Read the model definition and answer for the solid it produces. Units are mm, in the model's axes. Give positions to 0.01 mm unless a question says otherwise; leave off trailing zeros. Loops run counter-clockwise (first coordinate to the right, second up) from the corner with the lowest first, then second, coordinate; pieces in that order, holes last. Notation, with made-up numbers: (-36, 43.5) - (9, 43.5) arc R30 cw to (9, 69.5) - close; hole circle Ø11 at (69, 80.25). An arc over 180 degrees is marked (long way). Use a Markdown table: item, result. Add a question column.
Item 1: Consider probe 1 along X at (y, z) = (61.5, -12.25); probe 2 along X at (y, z) = (28, -13); probe 3 along Z at (x, y) = (4.5, 49). Determine where each line is inside the solid, lowest interval first. Write a range as [from, to].
Item 2: A cutting plane is placed at C-C (x = 0). Determine the outline of the cut face in (y, z).
Item 3: A cutting plane is placed at B-B (y = 37.5). Determine the outline of the cut face in (x, z).
Item 4: A cutting plane is placed at D-D (z = 12). Determine the outline of the cut face in (x, y), plus the area to 3 significant figures.
Item 5: A cutting plane is placed at A-A (z = 7). Determine the outline of the cut face in (x, y).
Autodesk Fusion 360 part; units mm, degrees
sketch "Sketch1" plane through (0, 0, 0) normal (0, 0, 1) x (1, 0, 0)
sketch "Sketch2" plane through (0, 0, 0) normal (0, 1, 0) x (1, 0, 0)
  line L0 (24, -15) -> (-24, -15)
  line L1 (-24, -15) -> (-24, 15)
  line L2 (-24, 15) -> (24, 15)
  line L3 (24, 15) -> (24, -15)
  line L4 (24, -15) -> (-24, 15) construction
  line L5 (-24, -15) -> (24, 15) construction
  dimension "d3" = 48
  dimension "d4" = 30
extrude "Extrude1" add sketch "Sketch2" along normal blind 80
sketch "Sketch3" plane through (0, 0, 0) normal (0, -1, 0) x (1, 0, 0)
  line L0 (-24, -15) -> (24, -15)
  line L1 (24, -15) -> (24, 15)
  line L2 (24, 15) -> (-24, 15)
  line L3 (-24, 15) -> (-24, -15)
  arc A0 (-12, 15) -> (12, 15) centre (0, 15) ccw
  arc A1 (12, -15) -> (-12, -15) centre (0, -15) ccw
  line L4 (-12, -15) -> (12, -15)
  line L5 (12, 15) -> (-12, 15)
  dimension "d7" = 12
  dimension "d8" = 12
extrude "Extrude2" cut sketch "Sketch3" against normal blind 80 contours L0 A1 L4 | L2 A0 L5
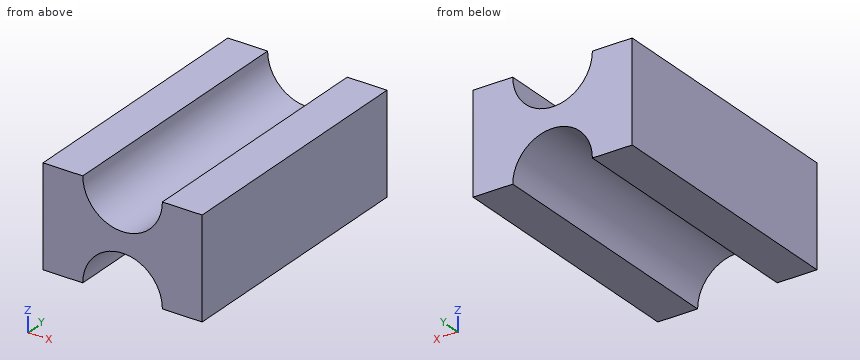
Geometry says:
| question | item | result |
|---|---|---|
| 1 | probe 1 | [-24, -11.68], [11.68, 24] |
| 1 | probe 2 | [-24, -11.83], [11.83, 24] |
| 1 | probe 3 | [-3.88, 3.88] |
| 2 | outline | (0, -3) - (80, -3) - (80, 3) - (0, 3) - close |
| 3 | outline | (-24, -15) - (-12, -15) arc R12 cw to (12, -15) - (24, -15) - (24, 15) - (12, 15) arc R12 cw to (-12, 15) - (-24, 15) - close |
| 4 | outline | (-24, 0) - (-11.62, 0) - (-11.62, 80) - (-24, 80) - close; (11.62, 0) - (24, 0) - (24, 80) - (11.62, 80) - close |
| 4 | area | 1,980 mm² |
| 5 | outline | (-24, 0) - (-8.94, 0) - (-8.94, 80) - (-24, 80) - close; (8.94, 0) - (24, 0) - (24, 80) - (8.94, 80) - close |
